Design review of the part built by this model. Coordinates are the model's own, in mm. A direction names the side the tool comes from. Give positions to 0.01 mm unless a question says otherwise; leave off trailing zeros. Loops run counter-clockwise (first coordinate to the right, second up) from the corner with the lowest first, then second, coordinate; pieces in that order, holes last. Notation, with made-up numbers: (-5.75, 12) - (16.25, 12) arc R23 cw to (16.25, 31) - close; hole circle Ø4 at (-33, 32). An arc over 180 degrees is marked (long way). One line per item, written item: value. Start each with the question number.
```python
from build123d import *

# Parameters (mm, degrees)
BOSS_EXTRUDE8_DEPTH   = 13
BOSS_EXTRUDE8_2_DEPTH = 13
SKETCH1_14_W          = 96.584344236
SKETCH1_14_H          = 25
BOSS_EXTRUDE9_DEPTH   = 15
BOSS_EXTRUDE10_DEPTH  = 9.5
EXTRUDE_THIN3_START   = -96
EXTRUDE_THIN3_DEPTH   = 96
FILLET1_R             = 2.5


# Read off the part's stored shape, not the designer's step: Extrude-Thin3
with BuildPart() as part:
    # Sketch1 → Boss-Extrude8 (new, symmetric)
    with BuildSketch(Plane(origin=(0, 0, 0), x_dir=(0, 0, -1), z_dir=(1, 0, 0))):
        Polygon((140, 48), (105, 48), (105, 31), (133, 31), (140, 38), align=None)
    extrude(amount=BOSS_EXTRUDE8_DEPTH, both=True)



with BuildPart() as body_2:
    # Sketch1 → Boss-Extrude8 2 (new, symmetric)
    with BuildSketch(Plane(origin=(0, 0, 0), x_dir=(0, 0, -1), z_dir=(1, 0, 0))):
        Polygon((105, -31), (105, -48), (140, -48), (140, -38), (133, -31), align=None)
    extrude(amount=BOSS_EXTRUDE8_2_DEPTH, both=True)


with BuildPart() as body_3:
    # Sketch1<14> → Boss-Extrude9 (new, symmetric)
    with BuildSketch(Plane(origin=(0, 0, 0), x_dir=(0, 0, -1), z_dir=(1, 0, 0))):
        with Locations((54.792172118, 0)):
            Rectangle(SKETCH1_14_W, SKETCH1_14_H)
    extrude(amount=BOSS_EXTRUDE9_DEPTH, both=True)


with BuildPart() as part_1:
    add(part.part)

    add(body_2.part)  # Boss-Extrude10 merges body 2

    add(body_3.part)  # Boss-Extrude10 merges body 3
    # Sketch1<15> → Boss-Extrude10 (add, symmetric)
    # profile 1 of 2: a face of its own
    with BuildSketch(Plane(origin=(0, 0, 0), x_dir=(0, 0, -1), z_dir=(1, 0, 0))):
        Polygon((6.5, 48), (6.5, 12.5), (103.084344236, 12.5), (114.5, 12.5), (133, 31), (105, 31), (105, 48), align=None)
        with BuildLine():
            ThreePointArc((30.5, 25), (25, 30.5), (30.5, 36))
            Line((30.5, 36), (81.5, 36))
            ThreePointArc((81.5, 36), (87, 30.5), (81.5, 25))
            Line((81.5, 25), (30.5, 25))
        make_face(mode=Mode.SUBTRACT)
    # profile 2 of 2: a face of its own
    with BuildSketch(Plane(origin=(0, 0, 0), x_dir=(0, 0, -1), z_dir=(1, 0, 0))):
        Polygon((6.5, -12.5), (6.5, -48), (105, -48), (105, -31), (133, -31), (114.5, -12.5), (103.084344236, -12.5), align=None)
        with BuildLine():
            Line((81.5, -36), (30.5, -36))
            ThreePointArc((30.5, -36), (25, -30.5), (30.5, -25))
            Line((30.5, -25), (81.5, -25))
            ThreePointArc((81.5, -25), (87, -30.5), (81.5, -36))
        make_face(mode=Mode.SUBTRACT)
    extrude(amount=BOSS_EXTRUDE10_DEPTH, both=True)

    # Extrude-Thin3 outline → Extrude-Thin3 (add)
    with BuildSketch(Plane(origin=(0, 48, 0), x_dir=(1, 0, 0), z_dir=(0, 1, 0)).offset(EXTRUDE_THIN3_START)):
        Polygon((-9.5, -0.104199667), (-3, -0.104199667), (-3, 0), (3.5, 0), (3.5, 6.5), (-9.5, 6.5), align=None)
    extrude(amount=EXTRUDE_THIN3_DEPTH)

    # Fillet1
    fillet1_edges = [part_1.edges().sort_by_distance(p)[0] for p in [
        (9.5, 30.5, -87),
        (9.5, 25, -56),
        (9.5, 30.5, -25),
        (-9.5, 36, -56),
        (9.5, 36, -56),
        (-9.5, 30.5, -87),
        (-9.5, 30.5, -25),
        (-9.5, 25, -56),
        (-9.5, -25, -56),
        (-9.5, -30.5, -87),
        (9.5, -36, -56),
        (-9.5, -30.5, -25),
        (9.5, -25, -56),
        (9.5, -30.5, -87),
        (9.5, -30.5, -25),
        (-9.5, -36, -56),
    ]]
    fillet(fillet1_edges, radius=FILLET1_R)


solid = part_1.part
```
(1) To check wall thickness, follow L1, parallel to Y at x = 4.5, z = -31; L2, parallel to Y at x = 10.25, z = -128; L3, parallel to Y at x = -5.75, z = -110. State the ranges of each line that lie inside material, in increasing order. Write a range as from..to.
(2) For pin 1 Ø18 at (y, z) = (-31, -46) entering from +X; pin 2 Ø6 at (x, z) = (-13, -68.5) entering from +Y; pin 3 Ø1.6 at (x, y) = (-12, -5) entering from +Z, all flat-tipped, find the tip position at first contact; note any pin that passes through.
(3) Machinability: for faces 5 (the flat face through (12, 12.5, -54)), 6 (the cylindrical face through (0.1, -30.6, -25)), 7 (the flat face through (-11, -31, -119)), 8 (the flat face through (3.5, -1, -3)), 9 (the flat face through (0, -25, -127)), which of the approach directions +Z, -Z, +X, -X, +Y, -Y give a long, thin tool a straight path to every point of the face, cutting with its end or side? Answer none if there is none.
(4) Take a section at A-A on z = -59. State the section outline as (x, y) points, and give its area (3 significant figures).
(5) Draft analysis for pull direction Z (two halves, no side actions). For faces 1 (the flat face through (0, 48, -71)), 2 (the flat face through (11, 40, -105)), 3 (the cylindrical face through (-0.1, 30.4, -25)), 4 (the cylindrical face through (-0.1, 30.6, -87)), state which applies: pulls with the +Z half, pulls with the -Z half, needs draft (parallel to the pull), parting line crosses it, or undercut.
(6) Take a section at C-C on y = 14. State the section outline as (x, z) points.
(7) Take a section at B-B on x = -11.25. State the section outline as (y, z) points, and give its area (3 significant figures).
Here are the results:
1. L1: -48..-36, -25..25, 36..48
1. L2: -48..-31, 31..48
1. L3: -48..-12.5, 12.5..48
2. pin 1: x = 9.5
2. pin 2: y = 12.5
2. pin 3: z = -6.5
3. face 5: +Z, -Z, +X, +Y
3. face 6: +X, -X
3. face 7: +Z, -Z, -X
3. face 8: +Z, +X, +Y, -Y
3. face 9: -Z, +X, -X
4. outline: (-15, -12.5) - (-9.5, -12.5) - (-9.5, -22.5) arc R2.5 ccw to (-7, -25) - (7, -25) arc R2.5 ccw to (9.5, -22.5) - (9.5, -12.5) - (15, -12.5) - (15, 12.5) - (9.5, 12.5) - (9.5, 22.5) arc R2.5 ccw to (7, 25) - (-7, 25) arc R2.5 ccw to (-9.5, 22.5) - (-9.5, 12.5) - (-15, 12.5) - close; (-9.5, -48) - (9.5, -48) - (9.5, -38.5) arc R2.5 ccw to (7, -36) - (-7, -36) arc R2.5 ccw to (-9.5, -38.5) - close; (-9.5, 38.5) arc R2.5 ccw to (-7, 36) - (7, 36) arc R2.5 ccw to (9.5, 38.5) - (9.5, 48) - (-9.5, 48) - close
4. area: 1,670 mm²
5. face 1: needs draft
5. face 2: pulls with the +Z half
5. face 3: undercut
5. face 4: undercut
6. outline: (-9.5, -116) - (9.5, -116) - (9.5, -6.5) - (3.5, -6.5) - (3.5, 0) - (-3, 0) - (-3, 0.1) - (-9.5, 0.1) - close
7. outline: (-48, -140) - (-38, -140) - (-31, -133) - (-31, -105) - (-48, -105) - close; (-12.5, -103.08) - (12.5, -103.08) - (12.5, -6.5) - (-12.5, -6.5) - close; (31, -133) - (38, -140) - (48, -140) - (48, -105) - (31, -105) - close
7. area: 3,560 mm²
